from build123d import *

# Parameters (mm, degrees)
SKETCH1_W           = 70
SKETCH1_H           = 150
BOSS_EXTRUDE1_DEPTH = 6
SKETCH2_W           = 70
SKETCH2_H           = 3.0237272
BOSS_EXTRUDE2_DEPTH = 6


with BuildPart() as part:
    # Sketch1 → Boss-Extrude1 (new body)
    with BuildSketch(Plane(origin=(0, 0, 0), x_dir=(1, 0, 0), z_dir=(0, 1, 0))):
        with Locations((35, 75)):
            Rectangle(SKETCH1_W, SKETCH1_H)
    extrude(amount=BOSS_EXTRUDE1_DEPTH)

    # Sketch2 → Boss-Extrude2 (add)
    with BuildSketch(Plane(origin=(0, 6, 0), x_dir=(1, 0, 0), z_dir=(0, 1, 0))):
        with Locations((35, 1.5118636)):
            Rectangle(SKETCH2_W, SKETCH2_H)
        with Locations((35, 10.69788065)):
            Rectangle(SKETCH2_W, SKETCH2_H)
        with Locations((35, 19.8838977)):
            Rectangle(SKETCH2_W, SKETCH2_H)
        with Locations((35, 29.06991475)):
            Rectangle(SKETCH2_W, SKETCH2_H)
        with Locations((35, 38.2559318)):
            Rectangle(SKETCH2_W, SKETCH2_H)
        with Locations((35, 47.44194885)):
            Rectangle(SKETCH2_W, SKETCH2_H)
        with Locations((35, 56.6279659)):
            Rectangle(SKETCH2_W, SKETCH2_H)
        with Locations((35, 65.81398295)):
            Rectangle(SKETCH2_W, SKETCH2_H)
        with Locations((35, 75)):
            Rectangle(SKETCH2_W, SKETCH2_H)
        with Locations((35, 84.18601705)):
            Rectangle(SKETCH2_W, SKETCH2_H)
        with Locations((35, 93.3720341)):
            Rectangle(SKETCH2_W, SKETCH2_H)
        with Locations((35, 102.55805115)):
            Rectangle(SKETCH2_W, SKETCH2_H)
        with Locations((35, 111.7440682)):
            Rectangle(SKETCH2_W, SKETCH2_H)
        with Locations((35, 120.93008525)):
            Rectangle(SKETCH2_W, SKETCH2_H)
        with Locations((35, 130.1161023)):
            Rectangle(SKETCH2_W, SKETCH2_H)
        with Locations((35, 139.30211935)):
            Rectangle(SKETCH2_W, SKETCH2_H)
        with Locations((35, 148.4881364)):
            Rectangle(SKETCH2_W, SKETCH2_H)
    extrude(amount=BOSS_EXTRUDE2_DEPTH)


solid = part.part
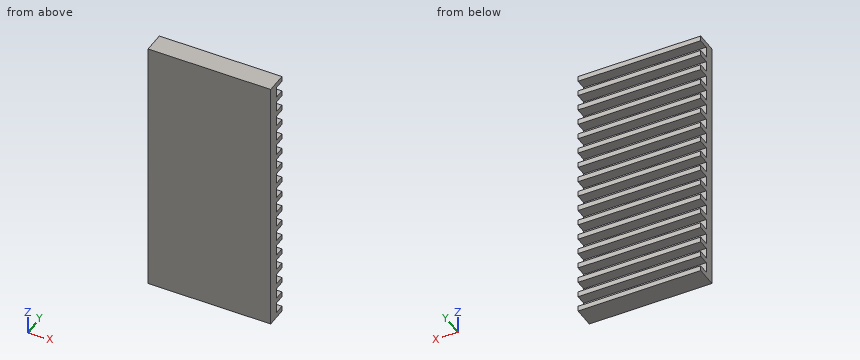
Model file for the job. Use its own axes, mm. Give positions to 0.01 mm unless a question says otherwise; leave off trailing zeros. Loops run counter-clockwise (first coordinate to the right, second up) from the corner with the lowest first, then second, coordinate; pieces in that order, holes last. Notation, with made-up numbers: (20, 82) -> (64, 82) arc R13 ccw to (64, 90) -> close; hole circle Ø9 at (80.5, -10). An arc over 180 degrees is marked (long way). Use a Markdown table: item, result. Add a question column.
(1) Slice it at A-A on y = 9. Give the number of separate pieces and of enclosed holes in the cut face, and give its area (3 significant figures).
(2) Drop flat-ended pins along their axis: pin 1 Ø5 at (y, z) = (10.5, -102.5) entering from -X; pin 2 Ø1.8 at (x, z) = (25, -125.5) entering from +Y. Give the stop position or say it passes through.
(3) Slice it at B-B on z = -117. List the corners of the cut face in (x, y), and give its area (3 significant figures).
(4) Wall check: line 1 along Y through (x, z) = (23.5, -34.5). Give the ranges that are in metal, low to high.
Filled sheet:
| question | item | result |
|---|---|---|
| 1 | separate pieces | 17 |
| 1 | enclosed holes | 0 |
| 1 | area | 3,600 mm2 |
| 2 | pin 1 | x = 0 |
| 2 | pin 2 | y = 6 |
| 3 | outline | (0, 0) -> (70, 0) -> (70, 6) -> (0, 6) -> close |
| 3 | area | 420 mm2 |
| 4 | line 1 | 0 to 6 |
